Check sheet for the modelled part. Datum: model origin and axes. Units: mm. Give positions to 0.01 mm unless a question says otherwise; leave off trailing zeros. Write each loop counter-clockwise with the first axis right and the second up, starting at its lowest first coordinate (ties: lowest second). Pieces come first, ordered by that corner, then holes. Notation, with made-up numbers: M 45.25,39.5 L 83.25,39.5 A26 cw 83.25,62.5 Z; hole C 67.25,-28.5 d4. An arc over 180 degrees is marked long. Write item = value, one per line. Start each with the question number.
1) Gauge pin test, flat ends, axial feed: pin 1 (1.8 mm diameter, centred on y = -4.5, z = -81, fed in from +X); pin 2 (1.8 mm diameter, centred on y = -4.5, z = -139.5, fed in from -X); pin 3 (3 mm diameter, centred on y = -2, z = 2.5, fed in from -X). Record the tip position at first contact, or that the pin passes through.
2) Sectioned sample at B-B, the plane x = 249.5. Record the cut outline in (y, z), then the cut area to 3 significant figures.
3) Sectioned sample at A-A, the plane z = -61. Record the cut outline in (x, y).
4) Sectioned sample at C-C, the plane z = -95. Count the separate pieces of the cut face and the enclosed holes in it, then the cut area to 3 significant figures.
5) Scan lines: L1, parallel to X at y = -0.5, z = -46; L2, parallel to X at y = -5.4, z = -58.5; L3, parallel to X at y = -0.95, z = -136.5. Record each from-to range of solid material in increasing order.
from build123d import *

# Parameters (mm, degrees)
F1_DEPTH = 6


with BuildPart() as f1:
    # F0 (on Front) → F1 (new body)
    with BuildSketch(Plane.XZ):
        Polygon((0, -121.23), (0, -144), (52, -144), (52, -137.99), (70.1, -137.99), (70.1, -144), (114, -144), (114, -137.99), (132.1, -137.99), (132.1, -144), (184, -144), (184, -71.99), (190.01, -71.99), (190.01, -144), (349.2, -144), (349.2, -71.99), (355.21, -71.99), (355.21, -144), (532.79, -144), (532.79, -71.99), (538.8, -71.99), (538.8, -144), (697.99, -144), (697.99, -71.99), (704, -71.99), (704, -144), (755.9, -144), (755.9, -137.99), (774, -137.99), (774, -144), (817.9, -144), (817.9, -137.99), (836, -137.99), (836, -144), (888, -144), (888, -121.23), (893.8, -121.23), (893.8, -119.23), (891, -117.23), (891, -107.23), (893.8, -105.23), (893.8, -103.23), (888, -103.23), (888, -53.21), (893.8, -53.21), (893.8, -51.21), (891, -49.21), (891, -39.21), (893.8, -37.21), (893.8, -35.21), (888, -35.21), (888, 0), (675, 0), (675, 5.8), (673, 5.8), (671, 3), (661, 3), (659, 5.8), (657, 5.8), (657, 0), (453, 0), (453, 5.8), (451, 5.8), (449, 3), (439, 3), (437, 5.8), (435, 5.8), (435, 0), (231, 0), (231, 5.8), (229, 5.8), (227, 3), (217, 3), (215, 5.8), (213, 5.8), (213, 0), (0, 0), (0, -35.21), (-5.8, -35.21), (-5.8, -37.21), (-3, -39.21), (-3, -49.21), (-5.8, -51.21), (-5.8, -53.21), (0, -53.21), (0, -103.23), (-5.8, -103.23), (-5.8, -105.23), (-3, -107.23), (-3, -117.23), (-5.8, -119.23), (-5.8, -121.23), align=None)
        with BuildLine():
            ThreePointArc((30, -35), (31.464466, -31.464466), (35, -30))
            Line((35, -30), (149, -30))
            ThreePointArc((149, -30), (152.535534, -31.464466), (154, -35))
            Line((154, -35), (154, -109))
            ThreePointArc((154, -109), (152.535534, -112.535534), (149, -114))
            Line((149, -114), (35, -114))
            ThreePointArc((35, -114), (31.464466, -112.535534), (30, -109))
            Line((30, -109), (30, -35))
        make_face(mode=Mode.SUBTRACT)
        with BuildLine():
            Line((220.01, -109), (220.01, -35))
            ThreePointArc((220.01, -35), (221.474466, -31.464466), (225.01, -30))
            Line((225.01, -30), (314.2, -30))
            ThreePointArc((314.2, -30), (317.735534, -31.464466), (319.2, -35))
            Line((319.2, -35), (319.2, -109))
            ThreePointArc((319.2, -109), (317.735534, -112.535534), (314.2, -114))
            Line((314.2, -114), (225.01, -114))
            ThreePointArc((225.01, -114), (221.474466, -112.535534), (220.01, -109))
        make_face(mode=Mode.SUBTRACT)
        with BuildLine():
            Line((385.21, -109), (385.21, -35))
            ThreePointArc((385.21, -35), (386.674466, -31.464466), (390.21, -30))
            Line((390.21, -30), (497.79, -30))
            ThreePointArc((497.79, -30), (501.325534, -31.464466), (502.79, -35))
            Line((502.79, -35), (502.79, -109))
            ThreePointArc((502.79, -109), (501.325534, -112.535534), (497.79, -114))
            Line((497.79, -114), (390.21, -114))
            ThreePointArc((390.21, -114), (386.674466, -112.535534), (385.21, -109))
        make_face(mode=Mode.SUBTRACT)
        with BuildLine():
            Line((568.8, -109), (568.8, -35))
            ThreePointArc((568.8, -35), (570.264466, -31.464466), (573.8, -30))
            Line((573.8, -30), (662.99, -30))
            ThreePointArc((662.99, -30), (666.525534, -31.464466), (667.99, -35))
            Line((667.99, -35), (667.99, -109))
            ThreePointArc((667.99, -109), (666.525534, -112.535534), (662.99, -114))
            Line((662.99, -114), (573.8, -114))
            ThreePointArc((573.8, -114), (570.264466, -112.535534), (568.8, -109))
        make_face(mode=Mode.SUBTRACT)
        with BuildLine():
            Line((734, -109), (734, -35))
            ThreePointArc((734, -35), (735.464466, -31.464466), (739, -30))
            Line((739, -30), (853, -30))
            ThreePointArc((853, -30), (856.535534, -31.464466), (858, -35))
            Line((858, -35), (858, -109))
            ThreePointArc((858, -109), (856.535534, -112.535534), (853, -114))
            Line((853, -114), (739, -114))
            ThreePointArc((739, -114), (735.464466, -112.535534), (734, -109))
        make_face(mode=Mode.SUBTRACT)
    extrude(amount=F1_DEPTH)


solid = f1.part
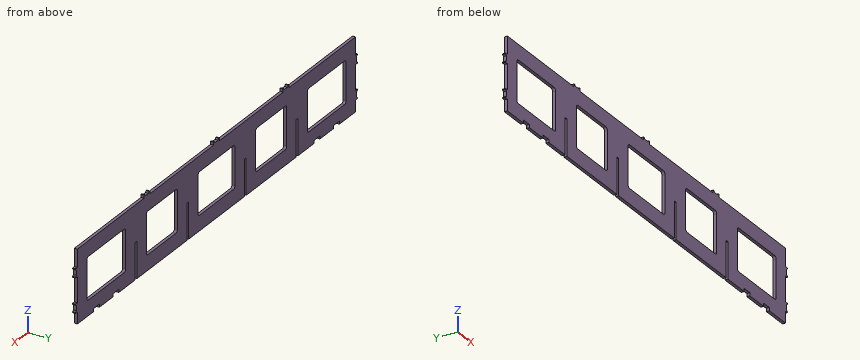
Data:
q1.pin_1 = 888
q1.pin_2 = 0
q1.pin_3 = 213
q2.outline = M -6,-144 L 0,-144 L 0,-114 L -6,-114 Z; M -6,-30 L 0,-30 L 0,0 L -6,0 Z
q2.area = 360 mm2
q3.outline = M 0,-6 L 30,-6 L 30,0 L 0,0 Z; M 154,-6 L 220.01,-6 L 220.01,0 L 154,0 Z; M 319.2,-6 L 385.21,-6 L 385.21,0 L 319.2,0 Z; M 502.79,-6 L 568.8,-6 L 568.8,0 L 502.79,0 Z; M 667.99,-6 L 734,-6 L 734,0 L 667.99,0 Z; M 858,-6 L 888,-6 L 888,0 L 858,0 Z
q4.separate_pieces = 10
q4.enclosed_holes = 0
q4.area = 1,800 mm2
q5.L1 = -3 to 30, 154 to 220.01, 319.2 to 385.21, 502.79 to 568.8, 667.99 to 734, 858 to 891
q5.L2 = 0 to 30, 154 to 220.01, 319.2 to 385.21, 502.79 to 568.8, 667.99 to 734, 858 to 888
q5.L3 = 0 to 184, 190.01 to 349.2, 355.21 to 532.79, 538.8 to 697.99, 704 to 888
